Autodesk Inventor part; units mm, degrees
ref_plane "YZ Plane" through (0, 0, 0) normal (1, 0, 0) x (0, 1, 0)
ref_plane "XZ Plane" through (0, 0, 0) normal (0, 1, 0) x (-1, 0, 0)
ref_plane "XY Plane" through (0, 0, 0) normal (0, 0, 1) x (1, 0, 0)
sketch "Sketch1" plane through (0, 0, 0) normal (0, 0, 1) x (1, 0, 0)
  line L0 (-7.3323, 0) -> (-3.6662, 6.35)
  line L1 (-3.6662, 6.35) -> (3.6662, 6.35)
  line L2 (3.6662, 6.35) -> (7.3323, 0)
  line L3 (7.3323, 0) -> (3.6662, -6.35)
  line L4 (3.6662, -6.35) -> (-3.6662, -6.35)
  line L5 (-3.6662, -6.35) -> (-7.3323, 0)
  point P0 (0, 0)
  point P1 (0, 0)
  dimension "d0" = 12.7
extrude "Pulley 1/2\" Hex" add sketch "Sketch1" along normal blind 25.4
sketch "Sketch2" plane through (0, 0, 25.4) normal (0, 0, 1) x (1, 0, 0)
  circle A0 centre (0, 0) radius 6.35
extrude "External 1/2\" Round" add sketch "Sketch2" along normal blind 7.9375
sketch "Sketch3" plane through (0, 0, 33.3375) normal (0, 0, 1) x (1, 0, 0)
  circle A0 centre (0, 0) radius 6.35
  line L0 (3.2748, 5.4404) -> (6.3489, 0.1158)
  line L1 (6.3489, -0.1158) -> (3.2748, -5.4404)
  line L2 (3.0742, -5.5563) -> (-3.0742, -5.5563)
  line L3 (-3.2748, -5.4404) -> (-6.3489, -0.1158)
  line L4 (-6.3489, 0.1158) -> (-3.2748, 5.4404)
  line L5 (-3.0742, 5.5563) -> (3.0742, 5.5563)
  dimension "d5" = 11.1125
extrude "Wheel 7/16\" Hex" add sketch "Sketch3" along normal blind 44.45 contours A0 L1 L2 L3 L4 L5 L0
sketch "Sketch4" plane through (0, 0, 77.7875) normal (0, 0, 1) x (1, 0, 0)
  arc A0 (-3.2748, -5.4404) -> (-3.0742, -5.5563) centre (0, 0) ccw
hole "Hole1" at (0, 0, 77.7875) direction (0, 0, -1) diameter 6.5278 end through all
properties part number "Center Axle" material "Aluminum 7075"
Design review of the part built by this model. Coordinates are the model's own, in mm. A direction names the side the tool comes from. Round coordinates to 2 decimals unless told otherwise and drop trailing zeros. Order: outer loops, then holes, each group sorted by start corner. A loop starts at its lowest first (then second) coordinate and runs counter-clockwise, first axis right, second up. Notation, with made-up numbers: (5.5, 20.25) - (54.5, 20.25) arc R16 cw to (54.5, 45.25) - close; hole circle Ø11 at (-10.5, 34). An arc over 180 degrees is marked (long way). Return JSON: item names as keys, results as strings.
Q1. Consider section B-B on y = 1.75. Write out the cut boundary in (x, z), plus the area to 3 significant figures.
Computed values:
{"outline": "(-6.32, 0) - (-2.76, 0) - (-2.76, 77.79) - (-5.41, 77.79) - (-5.41, 33.34) - (-6.1, 33.34) - (-6.1, 25.4) - (-6.32, 25.4) - close; (2.76, 0) - (6.32, 0) - (6.32, 25.4) - (6.1, 25.4) - (6.1, 33.34) - (5.41, 33.34) - (5.41, 77.79) - (2.76, 77.79) - close", "area": "470 mm2"}
Q2. For pin 1 Ø0.6 at (x, y) = (1, 6) entering from +Z; pin 2 Ø5 at (y, z) = (3, 59) entering from +X; pin 3 Ø3 at (x, z) = (4.5, 52) entering from -Y, all flat-tipped, find the tip position at first contact; note any pin that passes through.
Computed values:
{"pin 1": "stops at z = 33.34", "pin 2": "stops at x = 6.13", "pin 3": "stops at y = -5.56"}
Q3. Wall thickness on L1, parallel to Y at x = 0, z = 17; L2, parallel to Y at x = 0, z = 37.5: over which ranges is each line inside the solid? List them lowest first. Write a range as [from, to].
Computed values:
{"L1": "y = [-6.35, -3.26], [3.26, 6.35]", "L2": "y = [-5.56, -3.26], [3.26, 5.56]"}
Q4. The part is to be moulded in two halves that separate along Y. For faces 5 (the flat face through (-5.525, 3.131, 12.522)), 6 (the flat face through (-3, -6, 25.4)), 7 (the cylindrical face through (3.186, 0.708, 38.349)), say which applies: pulls with the +Y half, pulls with the -Y half, needs draft (parallel to the pull), parting line crosses it, or undercut.
Computed values:
{"face 5": "pulls with the +Y half", "face 6": "needs draft", "face 7": "undercut"}
Q5. Consider section A-A on x = -0.75. Write out the cut boundary in (y, z).
Computed values:
{"outline": "(-6.35, 0) - (-3.18, 0) - (-3.18, 77.79) - (-5.56, 77.79) - (-5.56, 33.34) - (-6.31, 33.34) - (-6.31, 25.4) - (-6.35, 25.4) - close; (3.18, 0) - (6.35, 0) - (6.35, 25.4) - (6.31, 25.4) - (6.31, 33.34) - (5.56, 33.34) - (5.56, 77.79) - (3.18, 77.79) - close"}
Q6. Machinability: for faces 1 (the flat face through (7, 0, 25.4)), 2 (the flat face through (-5, -3, 33.338)), 3 (the flat face through (-3, 6, 25.4)), 4 (the flat face through (0, -5.556, 55)), which of the approach directions +Z, -Z, +X, -X, +Y, -Y give a long, thin tool a straight path to every point of the face, cutting with its end or side? Answer none if there is none.
Computed values:
{"face 1": "+Z, +X", "face 2": "+Z, -X, -Y", "face 3": "+Z, -X, +Y", "face 4": "+Z, +X, -X, -Y"}
Q7. Consider section C-C on z = 70. Write out the cut boundary in (x, y).
Computed values:
{"outline": "(-6.35, -0.12) - (-3.27, -5.44) arc R6.35 ccw to (-3.07, -5.56) - (3.07, -5.56) arc R6.35 ccw to (3.27, -5.44) - (6.35, -0.12) arc R6.35 ccw to (6.35, 0.12) - (3.27, 5.44) arc R6.35 ccw to (3.07, 5.56) - (-3.07, 5.56) arc R6.35 ccw to (-3.27, 5.44) - (-6.35, 0.12) arc R6.35 ccw to start; hole circle Ø6.53 at (0, 0)"}
